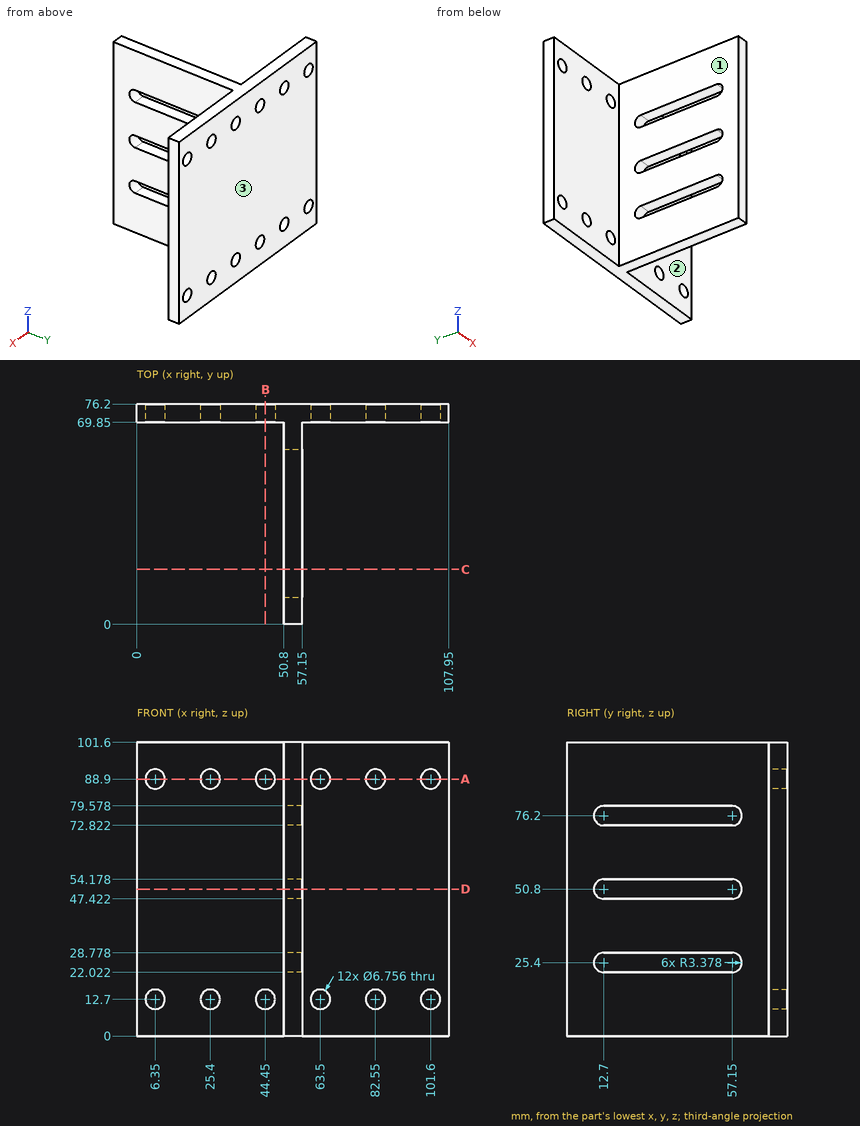
Here's the drawing with two shaded views (mm, measured from the low corner). I have some questions. A direction names the side the tool comes from. Round coordinates to 2 decimals unless told otherwise and drop trailing zeros. Loops run counter-clockwise (first coordinate to the right, second up) from the corner with the lowest first, then second, coordinate; pieces in that order, holes last. Notation, with made-up numbers: M 8,-9.5 L 40,-9.5 A9 cw 40,0.5 Z; hole C 22.25,53.25 d6. An arc over 180 degrees is marked long. Answer as CSV lines item,"result".
1) Which directions (+Z, -Z, +X, -X, +Y, -Y) give clear straight access to the entire face, cutting with the end or side of a thin tool? Please do the marked faces 1, 2 and 3.
From the geometry:
face 1,"+Z, -Z, -X, -Y"
face 2,"+Z, -Z, +X, -Y"
face 3,"+Z, -Z, +X, -X, +Y"
2) If I drill on probe 1 along Z at (x, y) = (44.45, 73); probe 2 along Z at (x, y) = (63, 74); probe 3 along X at (y, z) = (28, 35.5), over which ranges is the centre line in solid material (lowest first)?
From the geometry:
probe 1,"0 to 9.32, 16.08 to 85.52, 92.28 to 101.6"
probe 2,"0 to 9.36, 16.04 to 85.56, 92.24 to 101.6"
probe 3,"50.8 to 57.15"
3) Imagine slicing it at D-D on z = 50.8. List the corners of the cut face in (x, y) for me.
From the geometry:
outline,"M 0,69.85 L 50.8,69.85 L 50.8,60.53 L 57.15,60.53 L 57.15,69.85 L 107.95,69.85 L 107.95,76.2 L 0,76.2 Z; M 50.8,0 L 57.15,0 L 57.15,9.32 L 50.8,9.32 Z"
4) Imagine slicing it at C-C on y = 19. List the corners of the cut face in (x, z) for me.
From the geometry:
outline,"M 50.8,0 L 57.15,0 L 57.15,22.02 L 50.8,22.02 Z; M 50.8,28.78 L 57.15,28.78 L 57.15,47.42 L 50.8,47.42 Z; M 50.8,54.18 L 57.15,54.18 L 57.15,72.82 L 50.8,72.82 Z; M 50.8,79.58 L 57.15,79.58 L 57.15,101.6 L 50.8,101.6 Z"
5) Imagine slicing it at A-A on z = 88.9. Count the separate pieces of the cut face and the enclosed holes in it.
From the geometry:
separate pieces,"7"
enclosed holes,"0"
6) For pin 1 Ø10 at (y, z) = (19.5, 22) entering from +X; pin 2 Ø5 at (x, z) = (45, 17) entering from -Y, each with a flat end and sliding along its axis, tell me the tip position at first contact or that it passes through.
From the geometry:
pin 1,"x = 57.15"
pin 2,"y = 69.85"
7) Imagine slicing it at B-B on x = 44.45. List the corners of the cut face in (y, z) for me.
From the geometry:
outline,"M 69.85,0 L 76.2,0 L 76.2,9.32 L 69.85,9.32 Z; M 69.85,16.08 L 76.2,16.08 L 76.2,85.52 L 69.85,85.52 Z; M 69.85,92.28 L 76.2,92.28 L 76.2,101.6 L 69.85,101.6 Z"
